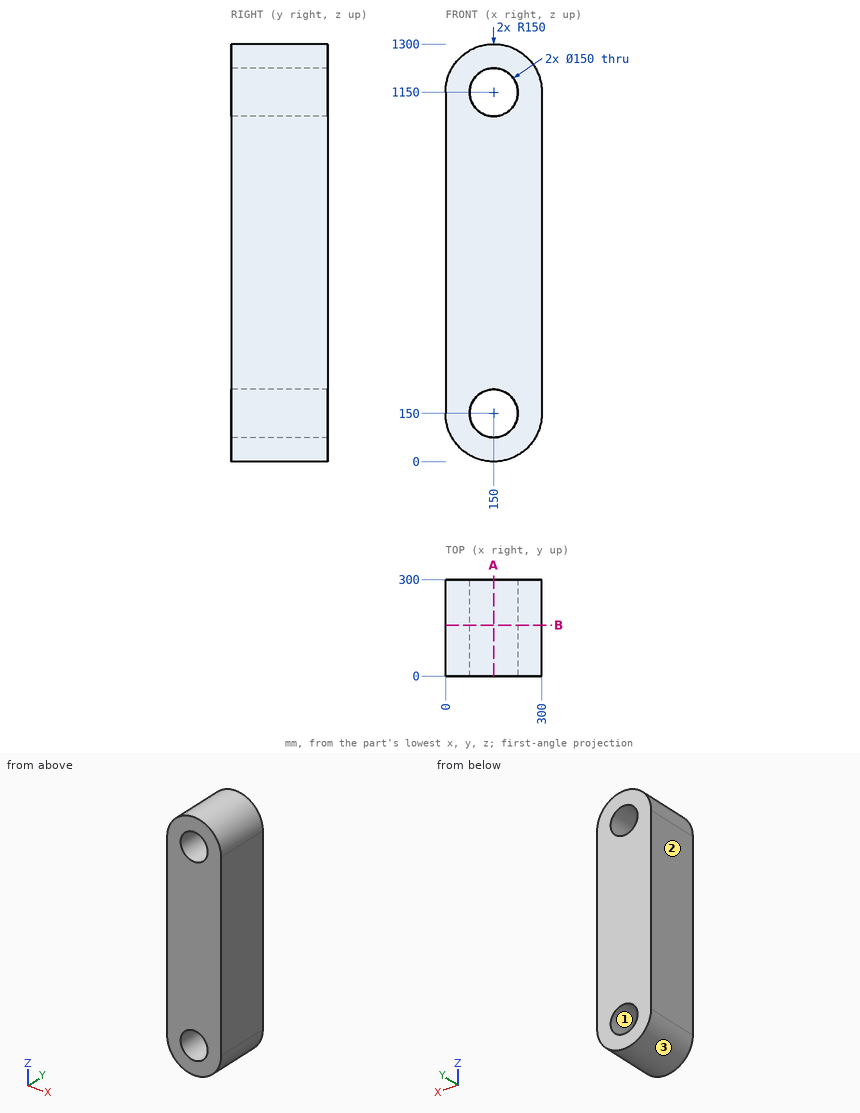
Drawing for the job (mm, zero at the part's lowest x, y, z). Give positions to 0.01 mm unless a question says otherwise; leave off trailing zeros. Write each loop counter-clockwise with the first axis right and the second up, starting at its lowest first coordinate (ties: lowest second). Pieces come first, ordered by that corner, then holes. Notation, with made-up numbers: (-17.75, 2.5) - (27.25, 2.5) arc R17 cw to (27.25, 21.5) - close; hole circle Ø1 at (87, 5.25). An arc over 180 degrees is marked (long way). Answer as CSV lines item,"result".
Q1. Band-saw the part on B-B (y = 158). Give the cut face in (x, z), and give its area (3 significant figures).
Result set:
outline,"(0, 150) arc R150 ccw to (300, 150) - (300, 1150) arc R150 ccw to (0, 1150) - close; hole circle Ø150 at (150, 150); hole circle Ø150 at (150, 1150)"
area,"335,000 mm²"
Q2. Band-saw the part on A-A (x = 150). Give the cut face in (y, z).
Result set:
outline,"(0, 0) - (300, 0) - (300, 75) - (0, 75) - close; (0, 225) - (300, 225) - (300, 1075) - (0, 1075) - close; (0, 1225) - (300, 1225) - (300, 1300) - (0, 1300) - close"
Q3. Pull direction Z, two halves, no side cores. Call the marked faces 1, 2 and 3: released by +Z, released by -Z, zero draft, split by the parting line, or undercut.
Result set:
face 1,"undercut"
face 2,"zero draft"
face 3,"released by -Z"
Q4. Drill centre lines: line 1 (Z direction, x = 150, y = 165); line 2 (X direction, y = 61, z = 1150); line 3 (Z direction, x = 208.5, y = 278.5). Where is each one in solid material? Low to high. Write a range as from..to.
Result set:
line 1,"0..75, 225..1075, 1225..1300"
line 2,"0..75, 225..300"
line 3,"11.88..103.07, 196.93..1103.07, 1196.93..1288.12"
Q5. Flat gauge pin, fed straight in: pin 1 Ø2 at (x, y) = (147.5, 188.5) entering from +Z. Where does the tip first touch, or does it go through?
Result set:
pin 1,"z = 1299.99"
